Check sheet for the modelled part. Datum: model origin and axes. Units: mm. A direction names the side the tool comes from. Coordinates: 2 decimals unless noted, no trailing zeros. Loops run counter-clockwise (first coordinate to the right, second up) from the corner with the lowest first, then second, coordinate; pieces in that order, holes last.
```python
from build123d import *

# Parameters (mm, degrees)
F0_W     = 232.602224
F0_H     = 218.396396
F1_DEPTH = 241.3
F2_R     = 50.8
F3_SIZE  = 50.8
F4_SIZE  = 50.8
F5_SIZE  = 50.8


with BuildPart() as f1:
    # F0 (on Front) → F1 (new body)
    with BuildSketch(Plane.XZ):
        Rectangle(F0_W, F0_H)
    extrude(amount=F1_DEPTH)

    # F2
    f2_edges = [f1.edges().sort_by_distance(p)[0] for p in [
        (116.301112, -120.65, 109.198198),
        (-116.301112, -120.65, 109.198198),
        (0, 0, 109.198198),
        (0, -241.3, 109.198198),
    ]]
    fillet(f2_edges, radius=F2_R)

    # F3
    f3_edges = [f1.edges().sort_by_distance(p)[0] for p in [
        (0, -241.3, -109.198198),
    ]]
    chamfer(f3_edges, length=F3_SIZE)

    # F4
    f4_edges = [f1.edges().sort_by_distance(p)[0] for p in [
        (-116.301112, -95.25, -109.198198),
    ]]
    chamfer(f4_edges, length=F4_SIZE)

    # F5
    f5_edges = [f1.edges().sort_by_distance(p)[0] for p in [
        (25.4, 0, -109.198198),
        (116.301112, -95.25, -109.198198),
    ]]
    chamfer(f5_edges, length=F5_SIZE)

    # F6: F1 across face


with BuildPart() as f1_1:
    add(f1.part)
    add(f1.part.mirror(Plane(origin=(116.301112, -120.65, 0), x_dir=(0, 1, 0), z_dir=(1, 0, 0))))

    # F7: F1 across face


with BuildPart() as f1_2:
    add(f1_1.part)
    add(f1_1.part.mirror(Plane(origin=(116.301112, 0, 0), x_dir=(1, 0, 0), z_dir=(0, 1, 0))))


solid = f1_2.part
```
1) Section check C-C on x = 226. Enter the section's corners in (y, z), plus the area to 3 significant figures.
Answer sheet:
outline: (-241.3, -58.4) - (-190.5, -109.2) - (-50.8, -109.2) - (0, -58.4) - (50.8, -109.2) - (190.5, -109.2) - (241.3, -58.4) - (241.3, 58.4) arc R50.8 ccw to (190.5, 109.2) - (50.8, 109.2) arc R50.8 ccw to (0, 58.4) arc R50.8 ccw to (-50.8, 109.2) - (-190.5, 109.2) arc R50.8 ccw to (-241.3, 58.4) - close
area: 98,000 mm2
2) Depth check by flat-ended pin: pin 1 (5 mm diameter, centred on y = 134, z = -71, fed in from +X); pin 2 (10 mm diameter, centred on y = -145, z = -71.5, fed in from -X); pin 3 (10 mm diameter, centred on x = 302.5, z = 69.5, fed in from +Y). Enter the tip coordinate at first touch or a pass-through.
Answer sheet:
pin 1: stops at x = 338.8
pin 2: stops at x = -108.2
pin 3: stops at y = 240.93
3) Section check D-D on z = -89.5. Enter the section's corners in (x, y).
Answer sheet:
outline: (-85.2, -210.2) - (85.2, -210.2) - (85.2, -31.1) - (-85.2, -31.1) - close; (-85.2, 31.1) - (85.2, 31.1) - (85.2, 210.2) - (-85.2, 210.2) - close; (147.4, -210.2) - (317.8, -210.2) - (317.8, -31.1) - (147.4, -31.1) - close; (147.4, 31.1) - (317.8, 31.1) - (317.8, 210.2) - (147.4, 210.2) - close
4) Section check A-A on y = -157. Enter the section's corners in (x, z), plus the area to 3 significant figures.
Answer sheet:
outline: (-116.3, -58.4) - (-65.5, -109.2) - (65.5, -109.2) - (116.3, -58.4) - (167.1, -109.2) - (298.1, -109.2) - (348.9, -58.4) - (348.9, 58.4) arc R50.8 ccw to (298.1, 109.2) - (167.1, 109.2) arc R50.8 ccw to (116.3, 58.4) arc R50.8 ccw to (65.5, 109.2) - (-65.5, 109.2) arc R50.8 ccw to (-116.3, 58.4) - close
area: 94,200 mm2
5) Scan lines: line 1 (X direction, y = 166, z = 68); line 2 (X direction, y = 139, z = -72); line 3 (Y direction, x = 287.5, z = 75.5). Record each from-to range of solid material in increasing order.
Answer sheet:
line 1: x = -115.39 to 115.39, 117.22 to 347.99
line 2: x = -102.7 to 102.7, 129.9 to 335.3
line 3: y = -238.33 to -2.97, 2.97 to 238.33
6) Set-up check for faces 4 (the flat face through (-1, 120, 109.198)), 5 (the flat face through (91.3, 119, -83.4)), 6 (the flat face through (234.2, -25.8, -84.2)): record each of +Z, -Z, +X, -X, +Y, -Y from which the full face is reachable in a straight line by a thin tool's end or side.
Answer sheet:
face 4: +Z, +X, -X, +Y, -Y
face 5: -Z, +Y, -Y
face 6: -Z, +X, -X
7) Mould release check, pull along X, two halves, no side actions. Record for faces 1 (the flat face through (141.346, -118.961, -83.443)), 2 (the flat face through (323.1, -119, -84.2)), 3 (the flat face through (-1, 120, -109.198)): +X half, -X half, draft (parallel to the pull), parting line (faces both ways), or undercut.
Answer sheet:
face 1: undercut
face 2: +X half
face 3: draft
8) Section check B-B on z = 89. Enter the section's corners in (x, y), plus the area to 3 significant figures.
Answer sheet:
outline: (-106.05, -231.05) - (106.05, -231.05) - (106.05, -10.25) - (-106.05, -10.25) - close; (-106.05, 10.25) - (106.05, 10.25) - (106.05, 231.05) - (-106.05, 231.05) - close; (126.55, -231.05) - (338.65, -231.05) - (338.65, -10.25) - (126.55, -10.25) - close; (126.55, 10.25) - (338.65, 10.25) - (338.65, 231.05) - (126.55, 231.05) - close
area: 187,000 mm2
